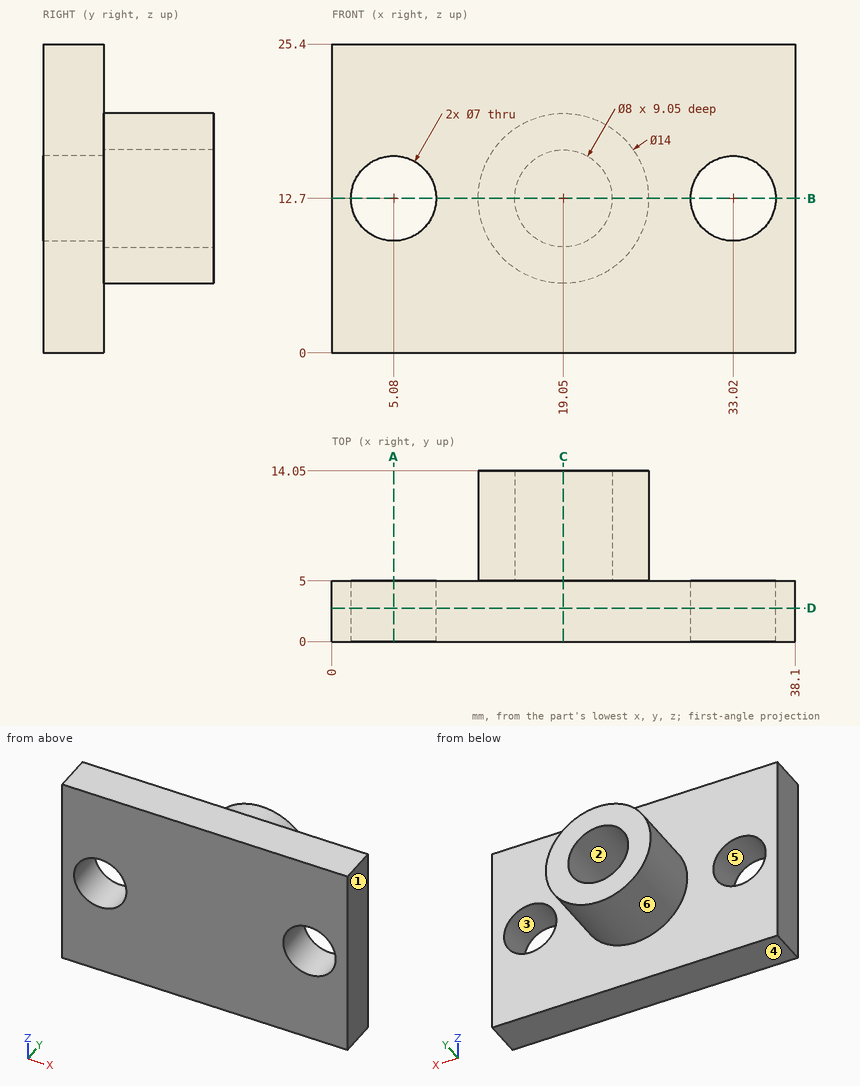
Verification items for this drawing (mm, ordinates from the low corner). A direction names the side the tool comes from. Round coordinates to 2 decimals unless told otherwise and drop trailing zeros. Order: outer loops, then holes, each group sorted by start corner. A loop starts at its lowest first (then second) coordinate and runs counter-clockwise, first axis right, second up. Notation, with made-up numbers: (71, 31) - (130, 31) arc R28 ccw to (130, 54) - close; hole circle Ø8 at (-15, 23). An arc over 180 degrees is marked (long way). Answer as CSV lines item,"result". Start each with the question number.
1) Section check A-A (x = 5.08). Record the cut outline in (y, z), then the cut area to 3 significant figures.
2) Section check D-D (y = 2.75). Record the cut outline in (x, z).
3) Draft check along X on the marked faces 3, 4, 5 and 6. Enter one of: +X half, -X half, draft (parallel to the pull), parting line (faces both ways), or undercut.
4) Scan lines: probe 1 along X at (y, z) = (3.4, 12.7); probe 2 along X at (y, z) = (7.75, 12.7); probe 3 along Y at (x, z) = (2.5, 15.25). Record each from-to range of solid material in increasing order.
5) Tool access check on the marked faces 1 and 2. Record the directions out of +Z, -Z, +X, -X, +Y, -Y that give a thin tool (end or side, any length) a straight path to the whole face; none if there is none.
6) Section check B-B (z = 12.7). Record the cut outline in (x, y), then the cut area to 3 significant figures.
7) Section check C-C (x = 19.05). Record the cut outline in (y, z), then the cut area to 3 significant figures.
8) Depth check by flat-ended pin: pin 1 (4 mm diameter, centred on x = 33.02, z = 12.7, fed in from -Y); pin 2 (1 mm diameter, centred on x = 29.5, z = 8, fed in from +Y). Enter the tip coordinate at first touch or a pass-through.
Determined:
1,outline,"(0, 0) - (5, 0) - (5, 9.2) - (0, 9.2) - close; (0, 16.2) - (5, 16.2) - (5, 25.4) - (0, 25.4) - close"
1,area,"92.0 mm^2"
2,outline,"(0, 0) - (38.1, 0) - (38.1, 25.4) - (0, 25.4) - close; hole circle Ø7 at (5.08, 12.7); hole circle Ø7 at (33.02, 12.7)"
3,face 3,"undercut"
3,face 4,"draft"
3,face 5,"undercut"
3,face 6,"parting line"
4,probe 1,"0 to 1.58, 8.58 to 29.52, 36.52 to 38.1"
4,probe 2,"12.05 to 15.05, 23.05 to 26.05"
4,probe 3,"0 to 5"
5,face 1,"+Z, -Z, +X, +Y, -Y"
5,face 2,"+Y"
6,outline,"(0, 0) - (1.58, 0) - (1.58, 5) - (0, 5) - close; (8.58, 0) - (29.52, 0) - (29.52, 5) - (26.05, 5) - (26.05, 14.05) - (23.05, 14.05) - (23.05, 5) - (15.05, 5) - (15.05, 14.05) - (12.05, 14.05) - (12.05, 5) - (8.58, 5) - close; (36.52, 0) - (38.1, 0) - (38.1, 5) - (36.52, 5) - close"
6,area,"175 mm^2"
7,outline,"(0, 0) - (5, 0) - (5, 5.7) - (14.05, 5.7) - (14.05, 8.7) - (5, 8.7) - (5, 16.7) - (14.05, 16.7) - (14.05, 19.7) - (5, 19.7) - (5, 25.4) - (0, 25.4) - close"
7,area,"181 mm^2"
8,pin 1,"through"
8,pin 2,"y = 5"
